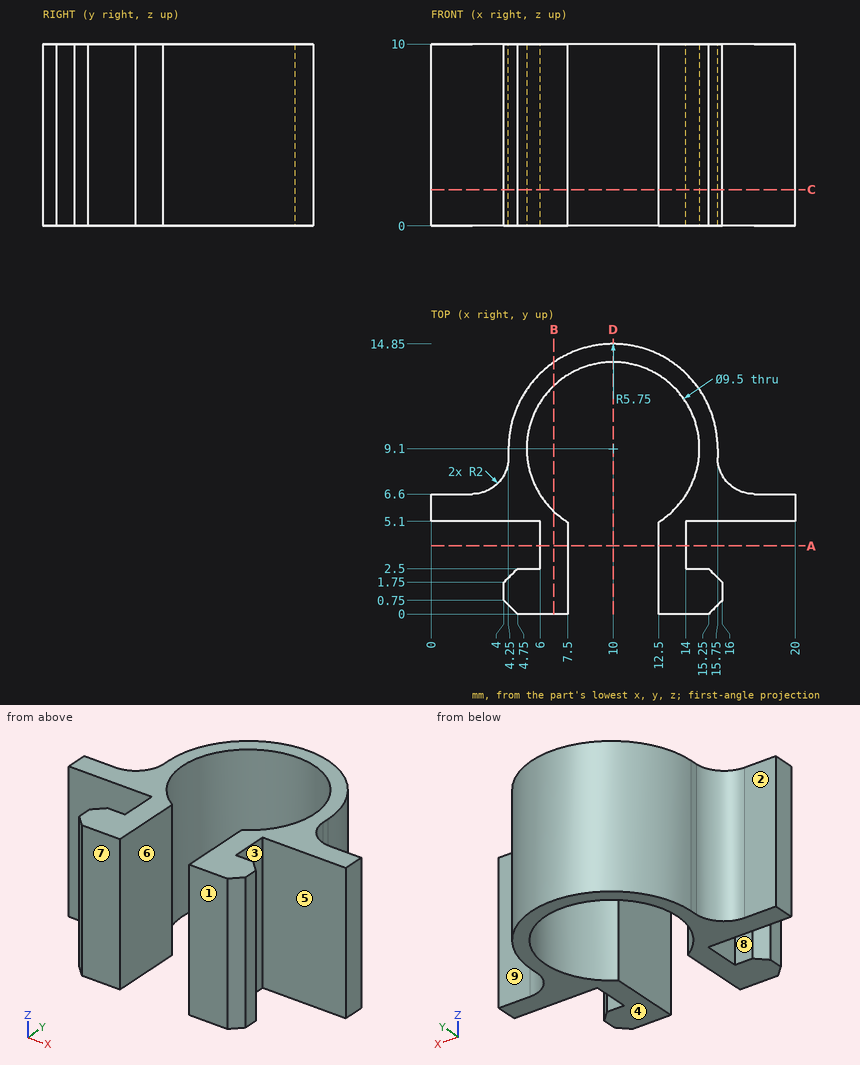
Print and shaded views of the part. All mm, measured from the part's lowest x, y and z. A direction names the side the tool comes from. Give positions to 0.01 mm unless a question says otherwise; leave off trailing zeros. Write each loop counter-clockwise with the first axis right and the second up, starting at its lowest first coordinate (ties: lowest second). Pieces come first, ordered by that corner, then holes. Notation, with made-up numbers: (66.5, 70.5) -> (83.5, 70.5) arc R27 cw to (83.5, 96.5) -> close; hole circle Ø3 at (42.5, -17.5). An arc over 180 degrees is marked (long way). Use CSV: the item, a comma, the result in double quotes. Start each with the question number.
1) Tool access for the marked faces 5, 6, 7, 8 and 9: list every direction of +Z, -Z, +X, -X, +Y, -Y with a clear straight run to the whole face (end or side of a thin tool).
2) Cut at C-C on z = 2. List the corners of the cut face in (x, y), plus the area to 3 significant figures.
3) Drill centre lines: L1, parallel to X at y = 4.75, z = 2.75; L2, parallel to X at y = 9.1, z = 7; L3, parallel to Y at x = 10, z = 3.75. Where is each one in solid material? Low to high.
4) Cut at A-A on y = 3.75. List the corners of the cut face in (x, z), plus the area to 3 significant figures.
5) Pin check, flat tips, straight feed: P1, Ø0.7, axis at x = 18.5, z = 6.5, coming from the +Y side; P2, Ø6, axis at x = 6, z = 7, coming from the -Y side; P3, Ø2.5, axis at y = 3.5, z = 4.5, coming from the -X side; P4, Ø1, axis at x = 17, z = 1.5, coming from the -Y side. Stop position of each tip, or through.
6) Cut at B-B on x = 6.75. List the corners of the cut face in (y, z).
7) Two-plate mould, pull along Y, no slides. Class the marked faces 1, 2, 3 and 4: released by +Y, released by -Y, zero draft, split by the parting line, or undercut.
8) Cut at D-D on x = 10. List the corners of the cut face in (y, z), plus the area to 4 significant figures.
Final values:
1,face 5,"+Z, -Z, +X"
1,face 6,"+Z, -Z, -Y"
1,face 7,"+Z, -Z, +X, -X, -Y"
1,face 8,"+Z, -Z, -X"
1,face 9,"+Z, -Z, +X, +Y"
2,outline,"(0, 5.1) -> (6, 5.1) -> (6, 2.5) -> (4.75, 2.5) -> (4, 1.75) -> (4, 0.75) -> (4.75, 0) -> (7.5, 0) -> (7.5, 5.06) arc R4.75 cw (long way) to (12.5, 5.06) -> (12.5, 0) -> (15.25, 0) -> (16, 0.75) -> (16, 1.75) -> (15.25, 2.5) -> (14, 2.5) -> (14, 5.1) -> (20, 5.1) -> (20, 6.6) -> (17.75, 6.6) arc R2 cw to (15.75, 8.6) -> (15.75, 9.1) arc R5.75 ccw to (4.25, 9.1) -> (4.25, 8.6) arc R2 cw to (2.25, 6.6) -> (0, 6.6) -> close"
2,area,"68.3 mm2"
3,L1,"x = 6 to 7.5, 12.5 to 14"
3,L2,"x = 4.25 to 5.25, 14.75 to 15.75"
3,L3,"y = 13.85 to 14.85"
4,outline,"(6, 0) -> (7.5, 0) -> (7.5, 10) -> (6, 10) -> close; (12.5, 0) -> (14, 0) -> (14, 10) -> (12.5, 10) -> close"
4,area,"30.0 mm2"
5,P1,"stops at y = 6.6"
5,P2,"stops at y = 0"
5,P3,"stops at x = 4.5"
5,P4,"stops at y = 5.1"
6,outline,"(0, 0) -> (5.64, 0) -> (5.64, 10) -> (0, 10) -> close; (12.56, 0) -> (13.84, 0) -> (13.84, 10) -> (12.56, 10) -> close"
7,face 1,"released by -Y"
7,face 2,"released by +Y"
7,face 3,"undercut"
7,face 4,"zero draft"
8,outline,"(13.85, 0) -> (14.85, 0) -> (14.85, 10) -> (13.85, 10) -> close"
8,area,"10.00 mm2"
